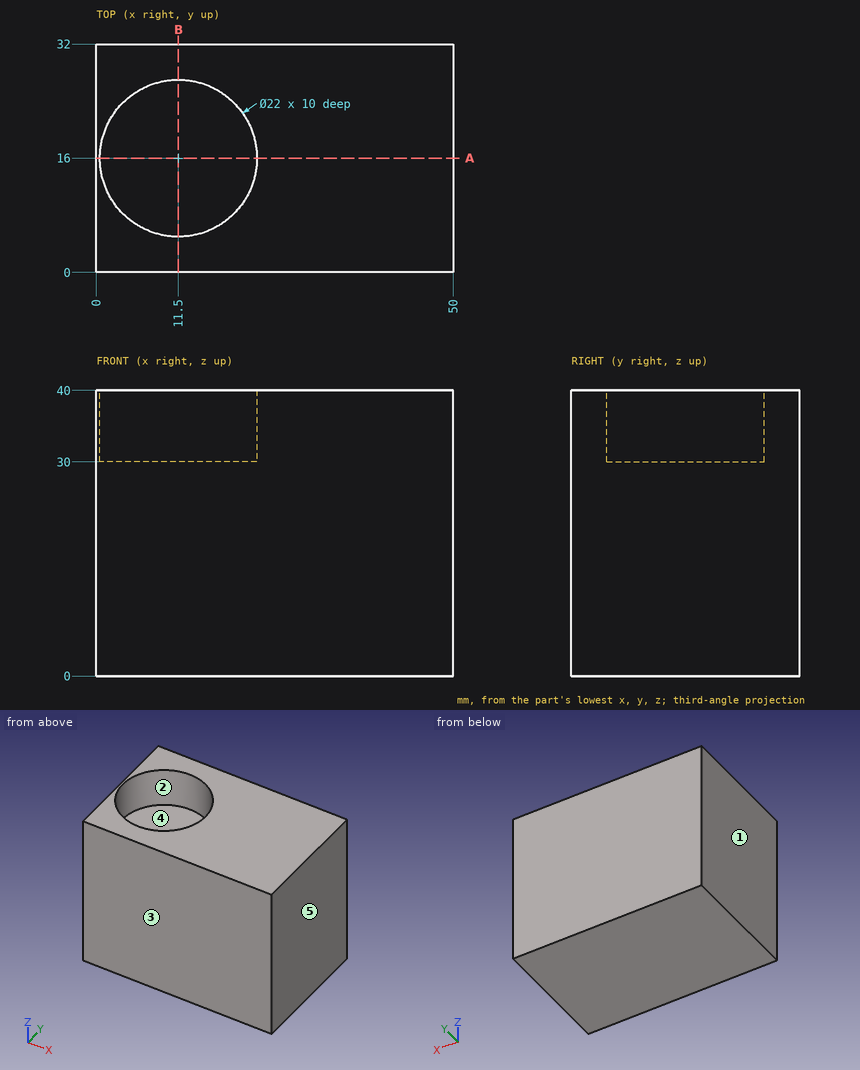
Study the drawing (mm; zero at the part's minimum x, y, z) and answer. A direction names the side the tool comes from. Round coordinates to 2 decimals unless told otherwise and drop trailing zeros. Loops run counter-clockwise (first coordinate to the right, second up) from the corner with the lowest first, then second, coordinate; pieces in that order, holes last. Notation, with made-up numbers: (74.25, 9) -> (119.25, 9) arc R10 ccw to (119.25, 14) -> close; hole circle Ø2 at (-9, -4.5). An arc over 180 degrees is marked (long way). One line per item, written item: value.
1) A cutting plane is placed at B-B (x = 11.5). Determine the outline of the cut face in (y, z), and give its area (3 significant figures).
Answer list:
outline: (0, 0) -> (32, 0) -> (32, 40) -> (27, 40) -> (27, 30) -> (5, 30) -> (5, 40) -> (0, 40) -> close
area: 1,060 mm²
2) For the marked faces 1 and 2, determine the directions among +Z, -Z, +X, -X, +Y, -Y from which every point of the face is accessible in a straight line to the end or side of a thin tool.
Answer list:
face 1: +Z, -Z, -X, +Y, -Y
face 2: +Z
3) Consider L1, parallel to X at y = 16, z = 38.25; L2, parallel to Y at x = 11.5, z = 37.5; L3, parallel to Z at x = 17, y = 21. Determine where each line is inside the solid, lowest interval first. Write a range as [from, to].
Answer list:
L1: x = [0, 0.5], [22.5, 50]
L2: y = [0, 5], [27, 32]
L3: z = [0, 30]
4) A flat-ended cylindrical pin translates along its axis: P1, Ø6.5, axis at x = 12.5, y = 12, coming from the +Z side. Find the tip coordinate at first contact, or state that the pin passes through.
Answer list:
P1: stops at z = 30
5) A cutting plane is placed at A-A (y = 16). Determine the outline of the cut face in (x, z).
Answer list:
outline: (0, 0) -> (50, 0) -> (50, 40) -> (22.5, 40) -> (22.5, 30) -> (0.5, 30) -> (0.5, 40) -> (0, 40) -> close
6) The mould has two halves that part along X. Classify the marked faces 3, 4 and 5: pulls with the +X half, pulls with the -X half, needs draft (parallel to the pull), parting line crosses it, or undercut.
Answer list:
face 3: needs draft
face 4: undercut
face 5: pulls with the +X half
